Verification items for the finished model (mm, model axes). Face numbers are marked on the shaded views. A direction names the side the tool comes from. Round coordinates to 2 decimals unless told otherwise and drop trailing zeros. Write each loop counter-clockwise with the first axis right and the second up, starting at its lowest first coordinate (ties: lowest second). Pieces come first, ordered by that corner, then holes. Notation, with made-up numbers: M 13.5,32 L 19.5,32 A27 ccw 19.5,48 Z; hole C 47.5,-11.5 d5. An arc over 180 degrees is marked long. One line per question, with ' | ' between items.
Autodesk Inventor part; units mm, degrees
ref_plane "YZ Plane" through (0, 0, 0) normal (1, 0, 0) x (0, 1, 0)
ref_plane "XZ Plane" through (0, 0, 0) normal (0, 1, 0) x (-1, 0, 0)
ref_plane "XY Plane" through (0, 0, 0) normal (0, 0, 1) x (1, 0, 0)
sketch "Sketch1" plane through (0, 0, 0) normal (0, 0, 1) x (1, 0, 0)
  line L0 (-7, -7) -> (7, -7)
  line L1 (7, -7) -> (7, 7)
  line L2 (7, 7) -> (-7, 7)
  line L3 (-7, 7) -> (-7, -7)
  line L4 (-7, -7) -> (7, 7) construction
  line L5 (7, -7) -> (-7, 7) construction
  point P0 (0, 0)
  dimension "d0" = 14
  dimension "d1" = 14
extrude "Plate1" add sketch "Sketch1" along normal blind 1
sketch "Sketch2" plane through (-6, 7, 1) normal (-1, 0, 0) x (0, -1, 0)
  line L0 (14, 0) -> (0, 0)
  line L1 (0, 0) -> (0, -15)
  line L2 (0, -15) -> (14, -15)
  line L3 (14, -15) -> (14, 0)
edge flange "Flange1" height 15 angle 90 thickness 1 bend radius 1 thickness toward (-1, 0, 0) relief tear relief width 1 relief depth 0.5 edges at (-7, 0, 0) wall of the first edge with corners at (-6, -7, 1) (-6, 7, 1) (-6, 7, -14) (-6, -7, -14)
bend "Bend1"
corner "Corner1"
sketch "Sketch3" plane through (0, 0, 1) normal (0, 0, 1) x (1, 0, 0)
  line L0 (7, -7) -> (7, 7)
  point P0 (0, 0)
  point P1 (1, 0)
  point P2 (7, 0)
  dimension "d13" = 6
hole "Hole1" at (1, 0, 1) direction (0, 0, -1) diameter 3 depth 1 tip angle 118
chamfer "Corner Chamfer1" distance 4 angle 45 2 edges at (7, 7, 0.5) (7, -7, 0.5)
equation "\"d1\" = d0"
equation "\"d19\" = Thickness"
equation "\"d3\" = BendReliefWidth"
equation "\"d4\" = BendReliefDepth"
equation "\"d5\" = MinimumRemnant"
equation "\"d6\" = BendRadius"
equation "\"d9\" = BendRadius"
equation "\"d10\" = CornerReliefSize"
equation "\"d11\" = GapSize"
equation "\"d12\" = JacobiRadiusSize"
equation "\"BendRadius\" = Thickness"
equation "\"BendReliefWidth\" = Thickness"
equation "\"BendReliefDepth\" = 0.5 * Thickness"
equation "\"CornerReliefSize\" = 4 * Thickness"
equation "\"MinimumRemnant\" = 2 * Thickness"
equation "\"TransitionRadius\" = BendRadius"
equation "\"JacobiRadiusSize\" = BendRadius"
equation "\"GapSize\" = Thickness"
equation "\"d2\" = BendRadius"
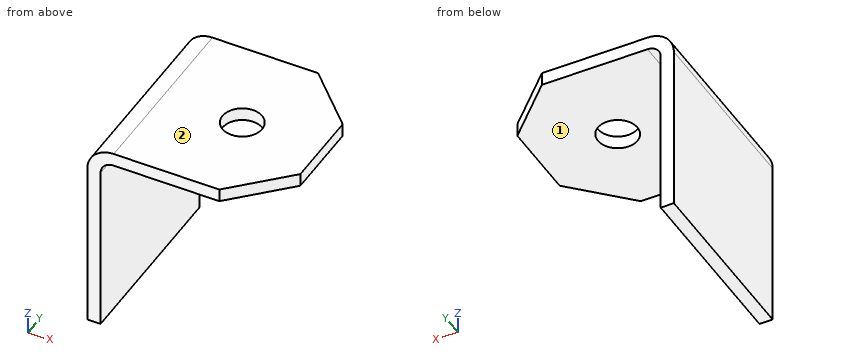
1. Section check C-C, the plane y = 4. Record the cut outline in (x, z).
Results:
outline: M -7,-14 L -6,-14 L -6,-1 A1 cw -5,0 L 6,0 L 6,1 L -5,1 A2 ccw -7,-1 Z
2. Go/stop test with flat-tipped pins: P1, Ø2, axis at y = 3, z = -9.5, coming from the +X side; P2, Ø6, axis at x = -3, z = -1, coming from the +Y side; P3, Ø3.5, axis at x = -0.5, y = -1.5, coming from the -Z side. Record where each tip stops, or that it passes through.
Results:
P1: stops at x = -6 | P2: stops at y = 7 | P3: stops at z = 0
3. Section check A-A, the plane y = 0. Record the cut outline in (x, z).
Results:
outline: M -7,-14 L -6,-14 L -6,-1 A1 cw -5,0 L -0.5,0 L -0.5,1 L -5,1 A2 ccw -7,-1 Z; M 2.5,0 L 7,0 L 7,1 L 2.5,1 Z
4. Tool access check on the marked faces 1 and 2. Record the directions out of +Z, -Z, +X, -X, +Y, -Y that give a thin tool (end or side, any length) a straight path to the whole face; none if there is none.
Results:
face 1: -Z, +X, +Y, -Y | face 2: +Z, +X, -X, +Y, -Y
5. Section check D-D, the plane x = 4.75. Record the cut outline in (y, z).
Results:
outline: M -5.25,0 L 5.25,0 L 5.25,1 L -5.25,1 Z
6. Section check B-B, the plane x = 1. Record the cut outline in (y, z), then the cut area to 3 significant figures.
Results:
outline: M -7,0 L -1.5,0 L -1.5,1 L -7,1 Z; M 1.5,0 L 7,0 L 7,1 L 1.5,1 Z | area: 11.0 mm2
7. Thickness scan on line 1 (Y direction, x = 1, z = 0.6); line 2 (Z direction, x = -1.25, y = 0); line 3 (X direction, y = -1, z = -7). Record the ranges inside material, lowest first.
Results:
line 1: y = -7 to -1.5, 1.5 to 7 | line 2: z = 0 to 1 | line 3: x = -7 to -6
